Source: CAD feature listing. Evaluate the final solid. Frame: model axes, mm. Face numbers are marked on the shaded views. A direction names the side the tool comes from. Give positions to 0.01 mm unless a question says otherwise; leave off trailing zeros. Write each loop counter-clockwise with the first axis right and the second up, starting at its lowest first coordinate (ties: lowest second). Pieces come first, ordered by that corner, then holes. Notation, with made-up numbers: M -9,0.25 L 25,0.25 A29 ccw 25,34.25 Z; hole C 71.5,35 d11. An arc over 180 degrees is marked long. Answer as a JSON object with one key per item and string values. Group by question number.
```python
from build123d import *

# Parameters (mm, degrees)
F1_DEPTH = 8
F3_R     = 3
F2_R     = 2.5
F4_DEPTH = 5.001
F5_R     = 2
F6_R     = 1


# Not quite as in the source:
# - a feature names something its author has since deleted; it is built from what else it names


with BuildPart() as f1:
    # F0 (on Top) → F1 (new body)
    with BuildSketch(Plane.XY):
        Polygon((0, 0), (0, 16.5), (-2, 16.5), (-2, -2), (22, -2), (22, 6.5), (3, 6.5), (3, 16.5), (1, 16.5), (1, 4.5), (20, 4.5), (20, 0), align=None)
    extrude(amount=-F1_DEPTH)

    # F3
    f3_edges = [f1.edges().sort_by_distance(p)[0] for p in [
        (-1, 16.5, 0),
        (-1, 16.5, -8),
        (2, 16.5, 0),
        (2, 16.5, -8),
    ]]
    fillet(f3_edges, radius=F3_R)

    # F2 (on face) → F4 (cut, through all)
    with BuildSketch(Plane.YZ.offset(3)):
        with Locations((11.5, -4)):
            Circle(F2_R)
    extrude(amount=-F4_DEPTH, mode=Mode.SUBTRACT)

    # F5
    f5_edges = [f1.edges().sort_by_distance(p)[0] for p in [
        (22, 6.5, -4),
        (22, -2, -4),
        (-2, -2, -4),
    ]]
    fillet(f5_edges, radius=F5_R)

    # F6
    f6_edges = [f1.edges().sort_by_distance(p)[0] for p in [
        (20, 4.5, -4),
        (20, 0, -4),
        (0, 0, -4),
        (1, 4.5, -4),
    ]]
    fillet(f6_edges, radius=F6_R)


solid = f1.part
```
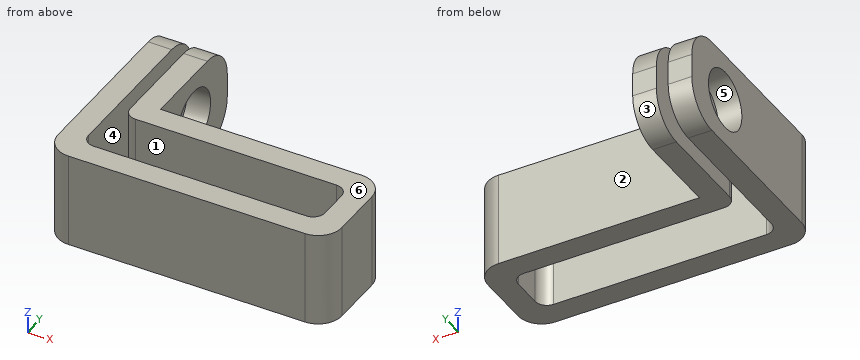
(1) Section C-C, the plane z = -4. Return loops of the section in (x, y).
(2) Pull-direction query (Z, two-part tool) for the marked faces 4, 5 and 6; classes: pulls with the +Z half, pulls with the -Z half, needs draft (parallel to the pull), parting line crosses it, or undercut.
(3) Section D-D, the plane z = -1. Return loops of the section in (x, y).
(4) Section A-A, the plane y = 11.5. Return loops of the section in (x, z), plus the area to 3 significant figures.
(5) Access query for the marked faces 1, 2 and 3. Directions: +Z, -Z, +X, -X, +Y, -Y. A direction counts if a zero-diameter tool reaches every point of the face in a straight line with its end or side. Return the directions, or none.
(6) Section B-B, the plane x = 5.75. Return loops of the section in (y, z), plus the area to 3 significant figures.
(7) Contact query for flat-ended pins moving along their axis: pin 1 Ø2.5 at (x, z) = (12.5, -5) entering from +Y; pin 2 Ø3 at (y, z) = (11.5, -4) entering from -X. Output: stop coordinate, or through.
(8) Ray query, L1, parallel to X at y = 11.25, z = -0.25; L2, parallel to X at y = 1.25, z = -2; L3, parallel to Z at x = 1.45, y = 11.5. Return the intervals inside material, ascending. Write a range as [from, to].
Reported:
{
 "1": {"outline": "M -2,0 A2 ccw 0,-2 L 20,-2 A2 ccw 22,0 L 22,4.5 A2 ccw 20,6.5 L 3,6.5 L 3,9 L 1,9 L 1,5.5 A1 ccw 2,4.5 L 19,4.5 A1 cw 20,3.5 L 20,1 A1 cw 19,0 L 1,0 A1 cw 0,1 L 0,9 L -2,9 Z; M -2,14 L 0,14 L 0,16.5 L -2,16.5 Z; M 1,14 L 3,14 L 3,16.5 L 1,16.5 Z"},
 "2": {"face 4": "needs draft", "face 5": "undercut", "face 6": "pulls with the +Z half"},
 "3": {"outline": "M -2,0 A2 ccw 0,-2 L 20,-2 A2 ccw 22,0 L 22,4.5 A2 ccw 20,6.5 L 3,6.5 L 3,15.74 L 1,15.74 L 1,5.5 A1 ccw 2,4.5 L 19,4.5 A1 cw 20,3.5 L 20,1 A1 cw 19,0 L 1,0 A1 cw 0,1 L 0,15.74 L -2,15.74 Z"},
 "4": {"outline": "M -2,-8 L 0,-8 L 0,-6.5 L -2,-6.5 Z; M -2,-1.5 L 0,-1.5 L 0,0 L -2,0 Z; M 1,-8 L 3,-8 L 3,-6.5 L 1,-6.5 Z; M 1,-1.5 L 3,-1.5 L 3,0 L 1,0 Z", "area": "12.0 mm2"},
 "5": {"face 1": "+Z, -Z", "face 2": "+Z, -Z, +X, +Y", "face 3": "-Z, +X, -X, +Y"},
 "6": {"outline": "M -2,-8 L 0,-8 L 0,0 L -2,0 Z; M 4.5,-8 L 6.5,-8 L 6.5,0 L 4.5,0 Z", "area": "32.0 mm2"},
 "7": {"pin 1": "stops at y = 6.5", "pin 2": "passes through"},
 "8": {"L1": "x = [-2, 0], [1, 3]", "L2": "x = [-2, 0], [20, 22]", "L3": "z = [-8, -6.5], [-1.5, 0]"}
}
